Could you check a few things on this drawing? It's one solid part, dimensions in mm from its lowest x, y, z. A direction names the side the tool comes from. Give positions to 0.01 mm unless a question says otherwise; leave off trailing zeros. Loops run counter-clockwise (first coordinate to the right, second up) from the corner with the lowest first, then second, coordinate; pieces in that order, holes last. Notation, with made-up numbers: (-32, 44.25) - (21, 44.25) arc R17 cw to (21, 68.25) - close; hole circle Ø6 at (23, 67.25). An arc over 180 degrees is marked (long way). Answer as a JSON object with one key per item and string values.
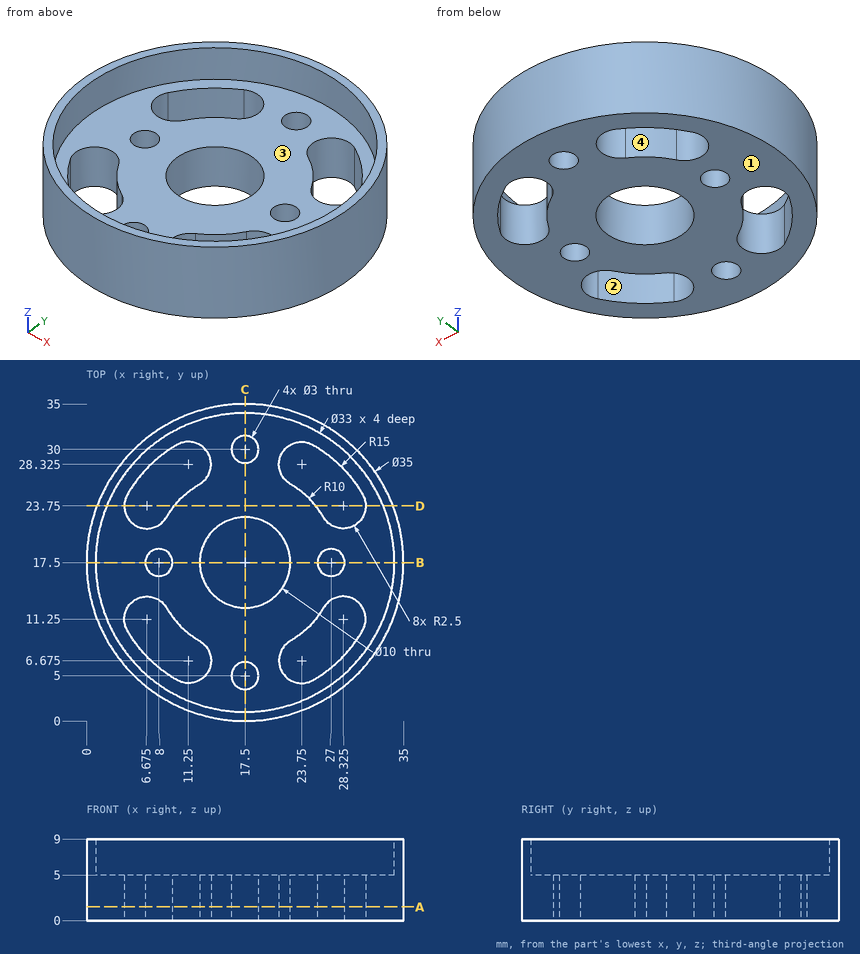
1) I need wall thicknesses on L1, parallel to Y at x = 17.5, z = 1.8; L2, parallel to Y at x = 27, z = 3; L3, parallel to X at y = 25, z = 3.75 (1 decimal). Which ranges of each line are inside material? Lowest first, please.
Check sheet entries:
{"L1": "0 to 3.5, 6.5 to 12.5, 22.5 to 28.5, 31.5 to 35", "L2": "2.8 to 5.89, 13.37 to 16, 19 to 21.63, 29.11 to 32.2", "L3": "1.7 to 4.5, 10.9 to 24.1, 30.5 to 33.3"}
2) I'm going to push flat-ended pins straight in: P1, Ø3.5, axis at x = 27, y = 17.5, coming from the +Z side; P2, Ø2.5, axis at x = 17.5, y = 30, coming from the +Z side; P3, Ø16.5, axis at x = 11.5, y = 24.5, coming from the +Z side; P4, Ø5, axis at y = 30.5, z = 2.5, coming from the +X side. Where does each tip first touch, or does it pass through?
Check sheet entries:
{"P1": "z = 5", "P2": "through", "P3": "z = 9", "P4": "x = 31.5"}
3) Imagine slicing it at B-B on y = 17.5. Write out the boundary of the cut face in (x, z).
Check sheet entries:
{"outline": "(0, 0) - (6.5, 0) - (6.5, 5) - (1, 5) - (1, 9) - (0, 9) - close; (9.5, 0) - (12.5, 0) - (12.5, 5) - (9.5, 5) - close; (22.5, 0) - (25.5, 0) - (25.5, 5) - (22.5, 5) - close; (28.5, 0) - (35, 0) - (35, 9) - (34, 9) - (34, 5) - (28.5, 5) - close"}
4) Imagine slicing it at A-A on z = 1.5. Give the number of separate pieces and of enclosed holes in the cut face, and give its area (3 significant figures).
Check sheet entries:
{"separate pieces": "1", "enclosed holes": "9", "area": "646 mm2"}
5) Imagine slicing it at C-C on x = 17.5. Write out the boundary of the cut face in (y, z).
Check sheet entries:
{"outline": "(0, 0) - (3.5, 0) - (3.5, 5) - (1, 5) - (1, 9) - (0, 9) - close; (6.5, 0) - (12.5, 0) - (12.5, 5) - (6.5, 5) - close; (22.5, 0) - (28.5, 0) - (28.5, 5) - (22.5, 5) - close; (31.5, 0) - (35, 0) - (35, 9) - (34, 9) - (34, 5) - (31.5, 5) - close"}
6) Which directions (+Z, -Z, +X, -X, +Y, -Y) give clear straight access to the entire face, cutting with the end or side of a thin tool? Please do the marked faces 3 and 4.
Check sheet entries:
{"face 3": "+Z", "face 4": "+Z, -Z"}
7) Imagine slicing it at D-D on y = 23.75. Write out the boundary of the cut face in (x, z) (1 decimal).
Check sheet entries:
{"outline": "(1.2, 0) - (4.2, 0) - (4.2, 5) - (2.2, 5) - (2.2, 9) - (1.2, 9) - close; (9.7, 0) - (25.3, 0) - (25.3, 5) - (9.7, 5) - close; (30.8, 0) - (33.8, 0) - (33.8, 9) - (32.8, 9) - (32.8, 5) - (30.8, 5) - close"}
8) If we mould it in two halves opening along Y, with no side actions, what happens to the marked faces 1 and 2? For each: released by +Y, released by -Y, zero draft, split by the parting line, or undercut.
Check sheet entries:
{"face 1": "zero draft", "face 2": "undercut"}
